```python
from build123d import *

# Parameters (mm, degrees)
SKETCH2_R                       = 39.243
BOSS_EXTRUDE1_DEPTH             = 6.35
SKETCH4_R                       = 39.243
SKETCH4_R_2                     = 36.5125
CUT_EXTRUDE1_DEPTH              = 3.175
F_1_4_0_25_DIAMETER_HOLE1_D     = 6.35
F_13_16_0_8125_DIAMETER_HOLE1_D = 20.6375
CUT_EXTRUDE3_DEPTH              = 3.175
SKETCH9_R                       = 6.0325
CUT_EXTRUDE2_DEPTH              = 1.5875


with BuildPart() as part:
    # Sketch2 → Boss-Extrude1 (new body)
    with BuildSketch(Plane(origin=(0, 0, 0), x_dir=(1, 0, 0), z_dir=(0, 1, 0))):
        Circle(SKETCH2_R)
    extrude(amount=BOSS_EXTRUDE1_DEPTH)

    # Sketch4 → Cut-Extrude1 (cut)
    with BuildSketch(Plane(origin=(0, 6.35, 0), x_dir=(1, 0, 0), z_dir=(0, 1, 0))):
        Circle(SKETCH4_R)
        Circle(SKETCH4_R_2, mode=Mode.SUBTRACT)
    extrude(amount=-CUT_EXTRUDE1_DEPTH, mode=Mode.SUBTRACT)

    # 1/4 (0.25) Diameter Hole1 (through all)
    with Locations(Plane(origin=(0, 6.35, 0), x_dir=(1, 0, 0), z_dir=(0, 1, 0))):
        with Locations((-17.960512242, 17.960512242), (-17.960512242, -17.960512242), (17.960512242, 17.960512242), (17.960512242, -17.960512242)):
            Hole(F_1_4_0_25_DIAMETER_HOLE1_D / 2)

    # 13/16 (0.8125) Diameter Hole1 (through all)
    with Locations(Plane(origin=(0, 6.35, 0), x_dir=(1, 0, 0), z_dir=(0, 1, 0))):
        with Locations((0, 0)):
            Hole(F_13_16_0_8125_DIAMETER_HOLE1_D / 2)

    # Sketch11 → Cut-Extrude3 (cut)
    with BuildSketch(Plane(origin=(0, 6.35, 0), x_dir=(1, 0, 0), z_dir=(0, 1, 0))):
        with BuildLine():
            Line((-5.601020514, 10.2), (5.601020514, 10.2))
            ThreePointArc((5.601020514, 10.2), (7.490842879, 10.570899501), (9.100291576, 11.628571429))
            ThreePointArc((9.100291576, 11.628571429), (11.914213562, 11.614213562), (11.928571429, 8.800291576))
            ThreePointArc((11.928571429, 8.800291576), (10.870899501, 7.190842879), (10.5, 5.301020514))
            Line((10.5, 5.301020514), (10.5, -25.901020514))
            ThreePointArc((10.5, -25.901020514), (10.870899501, -27.790842879), (11.928571429, -29.400291576))
            ThreePointArc((11.928571429, -29.400291576), (11.914213562, -32.214213562), (9.100291576, -32.228571429))
            ThreePointArc((9.100291576, -32.228571429), (7.490842879, -31.170899501), (5.601020514, -30.8))
            Line((5.601020514, -30.8), (-5.601020514, -30.8))
            ThreePointArc((-5.601020514, -30.8), (-7.490842879, -31.170899501), (-9.100291576, -32.228571429))
            ThreePointArc((-9.100291576, -32.228571429), (-11.914213562, -32.214213562), (-11.928571429, -29.400291576))
            ThreePointArc((-11.928571429, -29.400291576), (-10.870899501, -27.790842879), (-10.5, -25.901020514))
            Line((-10.5, -25.901020514), (-10.5, 5.301020514))
            ThreePointArc((-10.5, 5.301020514), (-10.870899501, 7.190842879), (-11.928571429, 8.800291576))
            ThreePointArc((-11.928571429, 8.800291576), (-11.914213562, 11.614213562), (-9.100291576, 11.628571429))
            ThreePointArc((-9.100291576, 11.628571429), (-7.490842879, 10.570899501), (-5.601020514, 10.2))
        make_face()
    extrude(amount=-CUT_EXTRUDE3_DEPTH, mode=Mode.SUBTRACT)

    # Sketch9 → Cut-Extrude2 (cut)
    with BuildSketch(Plane.XZ):
        with Locations((-17.960512242, 17.960512242)):
            Circle(SKETCH9_R)
        with Locations((17.960512242, 17.960512242)):
            Circle(SKETCH9_R)
        with Locations((17.960512242, -17.960512242)):
            Circle(SKETCH9_R)
        with Locations((-17.960512242, -17.960512242)):
            Circle(SKETCH9_R)
    extrude(amount=-CUT_EXTRUDE2_DEPTH, mode=Mode.SUBTRACT)


solid = part.part
```
The model under review builds one solid part; all positions refer to its coordinate system, in mm. A direction names the side the tool comes from. Give positions to 0.01 mm unless a question says otherwise; leave off trailing zeros. Order: outer loops, then holes, each group sorted by start corner. A loop starts at its lowest first (then second) coordinate and runs counter-clockwise, first axis right, second up. Notation, with made-up numbers: (-18.75, 19) - (20.25, 19) arc R20 ccw to (20.25, 54) - close; hole circle Ø8 at (-12, 34). An arc over 180 degrees is marked (long way). Use CSV: the item, a comma, the result in double quotes. Start each with the question number.
Q1. To check wall thickness, follow line 1 along Z through (x, y) = (0, 4.25); line 2 along X through (y, z) = (5.75, 19.5); line 3 along X through (y, z) = (5.5, 19). State the ranges of each line that lie inside material, in increasing order. Write a range as [from, to].
Q2. Tool access review of faces 4 (the cylindrical face through (20.48, 3.94, 19.89)), 5 (the cylindrical face through (-11.945, 4.785, -11.583)), 6 (the flat face through (-15, 1.588, -21)): name each direction out of +Z, -Z, +X, -X, +Y, -Y from which nothing blocks a thin tool from reaching the whole face with its end or side.
Q3. The part is to be moulded in two halves that separate along Z. For faces 1 (the cylindrical face through (-5.11, 1.57, -38.91)), 2 (the cylindrical face through (7.516, 4.785, 31.181)), 3 (the flat face through (8, 0, 8)), say which applies: +Z half, -Z half, draft (parallel to the pull), parting line (faces both ways), or undercut.
Q4. We need section B-B, the plane z = 3. Write out the cut boundary in (x, y) (3 decimals).
Q5. We need section D-D, the plane x = -28. Write out the cut boundary in (y, z) (3 decimals), and give its area (3 significant figures).
Q6. Clearance check with flat-ended pins moving along their axes: pin 1 Ø5 at (x, z) = (17.96, -17.96) entering from -Y; pin 2 Ø1 at (x, y) = (-16, 1) entering from -Z; pin 3 Ø1 at (y, z) = (5, 14.5) entering from +X; pin 4 Ø2.5 at (x, y) = (-0.5, 5.5) entering from -Z. State where each tip first meets the part, or that it passes through.
Q7. We need section C-C, the plane y = 5. State how many separate pieces and enclosed holes the cut face has, and give its area (3 significant figures).
Outcome:
1,line 1,"z = [-36.51, -10.32], [30.8, 36.51]"
1,line 2,"x = [-30.87, -20.74], [-15.18, -10.5], [10.5, 15.18], [20.74, 30.87]"
1,line 3,"x = [-31.18, -20.96], [-14.96, -10.5], [10.5, 14.96], [20.96, 31.18]"
2,face 4,"+Y, -Y"
2,face 5,"+Y"
2,face 6,"-Y"
3,face 1,"parting line"
3,face 2,"undercut"
3,face 3,"draft"
4,outline,"(-39.128, 0) - (-9.873, 0) - (-9.873, 3.175) - (-10.5, 3.175) - (-10.5, 6.35) - (-36.389, 6.35) - (-36.389, 3.175) - (-39.128, 3.175) - close; (9.873, 0) - (39.128, 0) - (39.128, 3.175) - (36.389, 3.175) - (36.389, 6.35) - (10.5, 6.35) - (10.5, 3.175) - (9.873, 3.175) - close"
5,outline,"(0, -27.496) - (3.175, -27.496) - (3.175, -23.434) - (6.35, -23.434) - (6.35, 23.434) - (3.175, 23.434) - (3.175, 27.496) - (0, 27.496) - close"
5,area,"323 mm^2"
6,pin 1,"passes through"
6,pin 2,"stops at z = -36.05"
6,pin 3,"stops at x = 33.72"
6,pin 4,"stops at z = -36.51"
7,separate pieces,"1"
7,enclosed holes,"5"
7,area,"3,150 mm^2"
